The listing builds one solid part. Answer for the finished solid, in the listing's coordinates (mm). A direction names the side the tool comes from. Coordinates: 2 decimals unless noted, no trailing zeros. Write each loop counter-clockwise with the first axis right and the second up, starting at its lowest first coordinate (ties: lowest second). Pieces come first, ordered by that corner, then holes. Notation, with made-up numbers: M 16,72 L 59,72 A21 cw 59,84 Z; hole C 73.5,77.25 d6. An arc over 180 degrees is marked long. Write item = value, one per line. Start each with the question number.
```python
from build123d import *

# Parameters (mm, degrees)
PAD_DEPTH = 13.8


with BuildPart() as part:
    # Sketch → Pad (new body)
    with BuildSketch(Plane.XZ):
        with BuildLine():
            Line((1, -0.4), (1, 0))
            Line((1, 0), (8, 0))
            add(Edge.make_bspline(
                [(18.65, 0), (16.551038, 0.042752), (14.664511, 0.25382), (13.32, 0.7), (11.950524, 0.264498), (9.995746, 0.073969), (8, 0)],
                knots=[0, 0, 0, 0, 0.25, 0.5, 0.75, 1, 1, 1, 1], degree=3))
            Line((18.65, 0), (28.65, 0))
            Line((28.65, 0), (28.65, -1.25))
            Line((28.65, -1.25), (18.65, -1.25))
            add(Edge.make_bspline(
                [(18.65, -1.25), (16.551038, -1.207248), (14.664511, -0.99618), (13.32, -0.55), (11.950524, -0.985502), (9.995746, -1.176031), (8, -1.25)],
                knots=[0, 0, 0, 0, 0.25, 0.5, 0.75, 1, 1, 1, 1], degree=3))
            Line((8, -1.25), (1, -1.65))
            Line((1, -1.65), (0, -1.707143))
            Line((0, -1.707143), (0, -0.4))
            Line((0, -0.4), (1, -0.4))
        make_face()
    extrude(amount=PAD_DEPTH)


solid = part.part
```
1. Each of these flat-tipped pins is pushed along its axis until it touches: pin 1 (3 mm diameter, centred on x = 23.5, y = -9, fed in from +Z); pin 2 (5 mm diameter, centred on x = 18, y = -11.5, fed in from +Z); pin 3 (6 mm diameter, centred on x = 25, y = -12, fed in from -Z). Where does it stop, or does it pass through?
2. The part is cut by section A-A, the plane x = 21.5. Write down the section's boundary in (y, z).
3. The part is cut by section B-B, the plane x = 6.25. Write down the section's boundary in (y, z).
4. Straight lines are drawn through the part: L1, parallel to X at y = -7.5, z = -0.25; L2, parallel to Z at x = 19.75, y = -2; L3, parallel to Z at x = 13.75, y = -1. For each, find the intervals that lie inside material, in ascending order. Write a range as [from, to].
5. For faces 1 (the face through (24, -7, -1.25)), 2 (the face through (28.65, -7, -1)), 3 (the face through (15, -13.8, 0)), 4 (the face through (0.5, -6.8, -0.4)), 5 (the face through (24, -7, 0)), determine the directions among +Z, -Z, +X, -X, +Y, -Y from which every point of the face is accessible in a straight line to the end or side of a thin tool.
Solution:
q1.pin_1 = 0
q1.pin_2 = 0.18
q1.pin_3 = -1.25
q2.outline = M -13.8,-1.25 L 0,-1.25 L 0,0 L -13.8,0 Z
q3.outline = M -13.8,-1.35 L 0,-1.35 L 0,0 L -13.8,0 Z
q4.L1 = [1, 28.65]
q4.L2 = [-1.25, 0]
q4.L3 = [-0.74, 0.51]
q5.face_1 = -Z, +X, +Y, -Y
q5.face_2 = +Z, -Z, +X, +Y, -Y
q5.face_3 = +Z, -Z, +X, -X, -Y
q5.face_4 = +Z, -X, +Y, -Y
q5.face_5 = +Z, +X, +Y, -Y
